Verification items for the finished model (mm, model axes). A direction names the side the tool comes from. Give positions to 0.01 mm unless a question says otherwise; leave off trailing zeros. Write each loop counter-clockwise with the first axis right and the second up, starting at its lowest first coordinate (ties: lowest second). Pieces come first, ordered by that corner, then holes. Notation, with made-up numbers: (2.25, 43.25) - (35.25, 43.25) arc R24 ccw to (35.25, 65.25) - close; hole circle Ø4 at (-34, -28.75). An arc over 180 degrees is marked (long way). Answer as a JSON object with one key per item and string values. Group by question number.
Item 1: Tool access check on faces 4 (the face through (66, 7, 2)), 5 (the face through (-66, 47, 2)), 6 (the face through (-64, -26, 1)), 7 (the face through (-1, -20, 0)). Record the directions out of +Z, -Z, +X, -X, +Y, -Y that give a thin tool (end or side, any length) a straight path to the whole face; none if there is none.
Item 2: Sectioned sample at D-D, the plane y = 40. Record the boundary of the cut face in (x, z), and give its area (3 significant figures).
Item 3: Draft check along Y on faces 1 (the face through (-40, -30, 2)), 2 (the face through (68.5, 49, 2)), 3 (the face through (-1, 51, 2)). Enter one of: +Y half, -Y half, draft (parallel to the pull), parting line (faces both ways), or undercut.
Item 4: Sectioned sample at B-B, the plane x = -53. Record the boundary of the cut face in (y, z).
Item 5: Sectioned sample at A-A, the plane y = -37.5. Record the boundary of the cut face in (x, z), and give its area (3 significant figures).
Item 6: Scan lines: line 1 along X through (y, z) = (-10, 0.25); line 2 along Y through (x, z) = (16.5, 0.75); line 3 along Y through (x, z) = (-25.5, -10.5). Record each from-to range of solid material in increasing order. Write a range as [from, to].
Item 7: Sectioned sample at C-C, the plane y = -6.5. Record the boundary of the cut face in (x, z).
Item 8: Go/stop test with flat-tipped pins: pin 1 (2 mm diameter, centred on y = 27.5, z = 0.5, fed in from +X); pin 2 (22.5 mm diameter, centred on x = 36.5, y = -29.5, fed in from -Z); pin 3 (1.2 mm diameter, centred on x = 65, z = 2, fed in from -Y); pin 4 (8 mm diameter, centred on x = 3.5, z = -1, fed in from +Y). Record where each tip stops, or that it passes through.
```python
from build123d import *

# Parameters (mm, degrees)
SKETCH1_W           = 137
SKETCH1_H           = 96
BOSS_EXTRUDE1_DEPTH = 4
SKETCH2_W           = 2.5
SKETCH2_H           = 40
SKETCH2_W_2         = 4.5
CUT_EXTRUDE1_DEPTH  = 4
SKETCH3_W           = 137
SKETCH3_H           = 4
BOSS_EXTRUDE2_DEPTH = 3
SKETCH4_W           = 137
SKETCH4_H           = 2
BOSS_EXTRUDE3_DEPTH = 11
SKETCH5_W           = 4.5
SKETCH5_H           = 8
CUT_EXTRUDE2_DEPTH  = 16
SKETCH6_W           = 39.2
SKETCH6_H           = 28.2
SKETCH6_W_2         = 69.2
SKETCH6_H_2         = 54.2
CUT_EXTRUDE3_DEPTH  = 2


with BuildPart() as part:
    # Sketch1 → Boss-Extrude1 (new body)
    with BuildSketch(Plane.XY):
        Rectangle(SKETCH1_W, SKETCH1_H)
    extrude(amount=BOSS_EXTRUDE1_DEPTH)

    # Sketch2 → Cut-Extrude1 (cut)
    with BuildSketch(Plane.XY.offset(4)):
        with Locations((-65.25, -20)):
            Rectangle(SKETCH2_W, SKETCH2_H)
        with Locations((65.25, -20)):
            Rectangle(SKETCH2_W, SKETCH2_H)
        with Locations((-66.25, 27)):
            Rectangle(SKETCH2_W_2, SKETCH2_H)
        with Locations((66.25, 27)):
            Rectangle(SKETCH2_W_2, SKETCH2_H)
    extrude(amount=-CUT_EXTRUDE1_DEPTH, mode=Mode.SUBTRACT)

    # Sketch3 → Boss-Extrude2 (add)
    with BuildSketch(Plane(origin=(0, 48, 0), x_dir=(1, 0, 0), z_dir=(0, 1, 0))):
        with Locations((0, -2)):
            Rectangle(SKETCH3_W, SKETCH3_H)
    extrude(amount=BOSS_EXTRUDE2_DEPTH)

    # Sketch4 → Boss-Extrude3 (add)
    with BuildSketch(Plane(origin=(0, 0, 0), x_dir=(-1, 0, 0), z_dir=(0, 0, -1))):
        with Locations((0, -47)):
            Rectangle(SKETCH4_W, SKETCH4_H)
    extrude(amount=BOSS_EXTRUDE3_DEPTH)

    # Sketch5 → Cut-Extrude2 (cut, through all)
    with BuildSketch(Plane.XY.offset(4)):
        with Locations((-66.25, -44)):
            Rectangle(SKETCH5_W, SKETCH5_H)
        with Locations((66.25, -44)):
            Rectangle(SKETCH5_W, SKETCH5_H)
    extrude(amount=-CUT_EXTRUDE2_DEPTH, mode=Mode.SUBTRACT)

    # Sketch6 → Cut-Extrude3 (cut)
    with BuildSketch(Plane(origin=(0, 0, 0), x_dir=(-1, 0, 0), z_dir=(0, 0, -1))):
        with Locations((-40.4, -30.2)):
            Rectangle(SKETCH6_W, SKETCH6_H)
        with Locations((40.4, -30.2)):
            Rectangle(SKETCH6_W, SKETCH6_H)
        with Locations((0, 17.8)):
            Rectangle(SKETCH6_W_2, SKETCH6_H_2)
    extrude(amount=-CUT_EXTRUDE3_DEPTH, mode=Mode.SUBTRACT)


solid = part.part
```
Geometry check:
{
 "1": {"face 4": "+Z, -Z, +X", "face 5": "+Z, -Z, -X", "face 6": "+Z, -Z, -Y", "face 7": "-Z, +X, -X, +Y"},
 "2": {"outline": "(-64, 0) - (-34.6, 0) - (-34.6, 2) - (34.6, 2) - (34.6, 0) - (64, 0) - (64, 4) - (-64, 4) - close", "area": "374 mm^2"},
 "3": {"face 1": "undercut", "face 2": "draft", "face 3": "+Y half"},
 "4": {"outline": "(-48, -11) - (-46, -11) - (-46, 0) - (-44.3, 0) - (-44.3, 2) - (-16.1, 2) - (-16.1, 0) - (51, 0) - (51, 4) - (-48, 4) - close"},
 "5": {"outline": "(-68.5, 0) - (-66.5, 0) - (-66.5, 4) - (-68.5, 4) - close; (-64, 0) - (-60, 0) - (-60, 2) - (-20.8, 2) - (-20.8, 0) - (20.8, 0) - (20.8, 2) - (60, 2) - (60, 0) - (64, 0) - (64, 4) - (-64, 4) - close; (66.5, 0) - (68.5, 0) - (68.5, 4) - (66.5, 4) - close", "area": "371 mm^2"},
 "6": {"line 1": "[-68.5, -66.5], [-64, 64], [66.5, 68.5]", "line 2": "[-48, -9.3], [44.9, 51]", "line 3": "[-48, -46]"},
 "7": {"outline": "(-68.5, 0) - (-66.5, 0) - (-66.5, 4) - (-68.5, 4) - close; (-64, 0) - (-34.6, 0) - (-34.6, 2) - (34.6, 2) - (34.6, 0) - (64, 0) - (64, 4) - (-64, 4) - close; (66.5, 0) - (68.5, 0) - (68.5, 4) - (66.5, 4) - close"},
 "8": {"pin 1": "x = 64", "pin 2": "z = 2", "pin 3": "y = 0", "pin 4": "y = 51"}
}
